```python
from build123d import *

# Parameters (mm, degrees)
SKETCH1_W                                = 56.2
SKETCH1_H                                = 134.9
SKETCH1_R                                = 2
BOSS_EXTRUDE1_DEPTH                      = 6.5
POLOLU_MOUNTING_BRACKET_R                = 2
POLOLU_37MM_MOUNTING_BRACKET_HOLES_DEPTH = 147.282945007
SKETCH2_R                                = 2
SPINDLE_MOUNT_DEPTH                      = 147.282945007


with BuildPart() as part:
    # Sketch1 → Boss-Extrude1 (new body)
    with BuildSketch(Plane(origin=(0, 0, 0), x_dir=(1, 0, 0), z_dir=(0, 1, 0))):
        with Locations((-28.1, 67.45)):
            Rectangle(SKETCH1_W, SKETCH1_H)
        with Locations(Location((-52.2, 104.9, 0), (0, 0, 90))):
            Circle(SKETCH1_R, mode=Mode.SUBTRACT)
        with Locations(Location((-4, 111.05, 0), (0, 0, 90))):
            Circle(SKETCH1_R, mode=Mode.SUBTRACT)
        with Locations(Location((-37, 80.8, 0), (0, 0, 90))):
            Circle(SKETCH1_R, mode=Mode.SUBTRACT)
        with Locations(Location((-52.2, 30, 0), (0, 0, 90))):
            Circle(SKETCH1_R, mode=Mode.SUBTRACT)
        with Locations(Location((-4, 28.7, 0), (0, 0, 90))):
            Circle(SKETCH1_R, mode=Mode.SUBTRACT)
    extrude(amount=BOSS_EXTRUDE1_DEPTH)

    # Pololu Mounting Bracket → Pololu 37mm mounting bracket holes (cut, through all)
    with BuildSketch(Plane(origin=(0, 6.5, 0), x_dir=(1, 0, 0), z_dir=(0, 1, 0))):
        with Locations(Location((-43.7, 4, 0), (0, 0, 270))):
            Circle(POLOLU_MOUNTING_BRACKET_R)
        with Locations(Location((-12.5, 4, 0), (0, 0, 270))):
            Circle(POLOLU_MOUNTING_BRACKET_R)
        with Locations(Location((-43.7, 42.4, 0), (0, 0, 270))):
            Circle(POLOLU_MOUNTING_BRACKET_R)
        with Locations(Location((-12.5, 42.4, 0), (0, 0, 270))):
            Circle(POLOLU_MOUNTING_BRACKET_R)
        with Locations(Location((-43.7, 130.9, 0), (0, 0, 270))):
            Circle(POLOLU_MOUNTING_BRACKET_R)
        with Locations(Location((-12.5, 130.9, 0), (0, 0, 270))):
            Circle(POLOLU_MOUNTING_BRACKET_R)
        with Locations(Location((-12.5, 92.5, 0), (0, 0, 270))):
            Circle(POLOLU_MOUNTING_BRACKET_R)
        with Locations(Location((-43.7, 92.5, 0), (0, 0, 270))):
            Circle(POLOLU_MOUNTING_BRACKET_R)
    extrude(amount=-POLOLU_37MM_MOUNTING_BRACKET_HOLES_DEPTH, mode=Mode.SUBTRACT)

    # Sketch2 → Spindle Mount (cut, through all)
    with BuildSketch(Plane.XZ):
        with Locations(Location((-24, -67.45, 0), (0, 0, 270))):
            Circle(SKETCH2_R)
        with Locations(Location((-10, -77.39530997, 0), (0, 0, 270))):
            Circle(SKETCH2_R)
        with Locations(Location((-10, -57.39530997, 0), (0, 0, 270))):
            Circle(SKETCH2_R)
    extrude(amount=-SPINDLE_MOUNT_DEPTH, mode=Mode.SUBTRACT)


solid = part.part
```
Build history of the part. All positions in model axes, mm. Round coordinates to 2 decimals unless told otherwise and drop trailing zeros. Loops run counter-clockwise (first coordinate to the right, second up) from the corner with the lowest first, then second, coordinate; pieces in that order, holes last.
Item 1: Saw through at D-D (x = -24). List the corners of the cut face in (y, z).
Item 2: Pin check, flat tips, straight feed: P1, Ø3, axis at x = -37, z = -80.8, coming from the -Y side; P2, Ø4.5, axis at x = -4, z = -28.7, coming from the +Y side. Stop position of each tip, or through.
Item 3: Saw through at B-B (x = -52.2). List the corners of the cut face in (y, z), then the cut area to 3 significant figures.
Item 4: Drill centre lines: line 1 along X through (y, z) = (4, -42.4); line 2 along X through (y, z) = (1.5, -67.45); line 3 along Z through (x, y) = (-13, 2.75). Where is each one in solid material? Low to high.
Item 5: Two-plate mould, pull along X, no slides. Class faces 1 (the face through (-28, 3, -134.9)), 2 (the face through (-42.348, 3.296, -132.374)), 3 (the face through (0, 3, -67)): released by +X, released by -X, zero draft, split by the parting line, or undercut.
Item 6: Saw through at A-A (z = -130.9). List the corners of the cut face in (x, y), then the cut area to 3 significant figures.
Item 7: Saw through at C-C (y = 3). State how many separate pieces and enclosed holes the cut face has, then the cut area to 3 significant figures.
Worked answers:
1. outline: (0, -134.9) - (6.5, -134.9) - (6.5, -69.45) - (0, -69.45) - close; (0, -65.45) - (6.5, -65.45) - (6.5, 0) - (0, 0) - close
2. P1: passes through
2. P2: stops at y = 6.5
3. outline: (0, -134.9) - (6.5, -134.9) - (6.5, -106.9) - (0, -106.9) - close; (0, -102.9) - (6.5, -102.9) - (6.5, -32) - (0, -32) - close; (0, -28) - (6.5, -28) - (6.5, 0) - (0, 0) - close
3. area: 825 mm2
4. line 1: x = -56.2 to -45.7, -41.7 to -14.5, -10.5 to 0
4. line 2: x = -56.2 to -26, -22 to 0
4. line 3: z = -134.9 to -132.84, -128.96 to -94.44, -90.56 to -44.34, -40.46 to -5.94, -2.06 to 0
5. face 1: zero draft
5. face 2: undercut
5. face 3: released by +X
6. outline: (-56.2, 0) - (-45.7, 0) - (-45.7, 6.5) - (-56.2, 6.5) - close; (-41.7, 0) - (-14.5, 0) - (-14.5, 6.5) - (-41.7, 6.5) - close; (-10.5, 0) - (0, 0) - (0, 6.5) - (-10.5, 6.5) - close
6. area: 313 mm2
7. separate pieces: 1
7. enclosed holes: 16
7. area: 7,380 mm2
